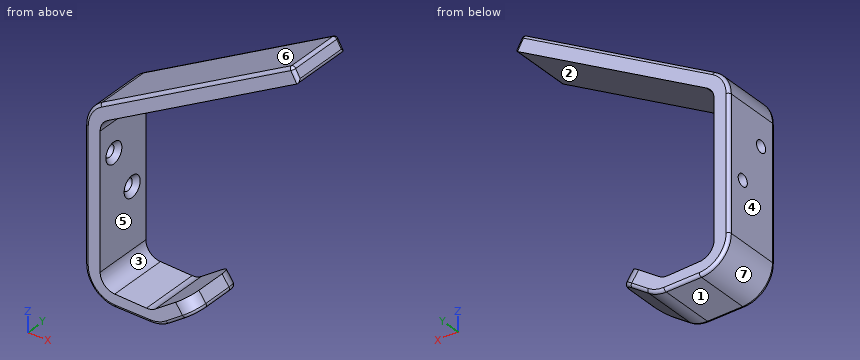
from build123d import *

# Parameters (mm, degrees)
F1_DEPTH       = 20
F2_R           = 10
F3_R           = 10
F4_R           = 5
F5_R           = 5
F6_R           = 5
F8_D           = 4
F8_DEPTH       = 12
F8_CSINK_D     = 7
F8_CSINK_ANGLE = 90
F8_TIP         = 1.2017212381
F9_T1_DEPTH    = 30.0048285071
F10_R          = 1
F11_T1_DEPTH   = 25
F11_T3_DEPTH   = 18
F11_T5_DEPTH   = 6.5
F11_T8_ANGLE   = 90
F11_T10_ANGLE  = 90


# Not quite as in the source:
# - a fillet or chamfer that OpenCascade refuses, or shapes differently, is made with other operations: its cross-section is extruded or revolved along the edge and cut away or added


with BuildPart() as f1:
    # F0 (on Front) → F1 (new body)
    with BuildSketch(Plane.XZ):
        Polygon((13.3003787555, -46.1032405242), (38.3003787555, -46.1032405242), (50.5316518247, -37.4287553132), (47.6391971652, -33.3503112419), (35.4933471628, -41.9642139506), (18.3003787555, -41.5471586402), (18.3003787555, 11.0100081298), (85.0824110582, 49.5666324568), (82.5824110582, 53.8967594758), (13.3003787555, 13.8967594758), align=None)
    extrude(amount=F1_DEPTH)

    # F2
    f2_edges = [f1.edges().sort_by_distance(p)[0] for p in [
        (13.300379, -10, 13.896759),
        (13.300379, -10, -46.103241),
    ]]
    fillet(f2_edges, radius=F2_R)

    # F3
    f3_edges = [f1.edges().sort_by_distance(p)[0] for p in [
        (38.300379, -10, -46.103241),
    ]]
    fillet(f3_edges, radius=F3_R)

    # F4
    f4_edges = [f1.edges().sort_by_distance(p)[0] for p in [
        (18.300379, -10, 11.010008),
    ]]
    fillet(f4_edges, radius=F4_R)

    # F5
    f5_edges = [f1.edges().sort_by_distance(p)[0] for p in [
        (18.300379, -10, -41.547159),
    ]]
    fillet(f5_edges, radius=F5_R)

    # F6
    f6_edges = [f1.edges().sort_by_distance(p)[0] for p in [
        (35.493347, -10, -41.964214),
    ]]
    fillet(f6_edges, radius=F6_R)

    # F8
    with Locations(Plane.YZ.offset(18.3003787555)):
        with Locations((-6, -16.6669744052), (-14, -1.8767432161)):
            CounterSinkHole(F8_D / 2, F8_CSINK_D / 2, depth=F8_DEPTH, counter_sink_angle=F8_CSINK_ANGLE)
            with Locations((0, 0, -(F8_DEPTH + F8_TIP / 2))):  # 118° drill point
                Cone(0, F8_D / 2, F8_TIP, mode=Mode.SUBTRACT)

    # F9: fillet of radius 5 on 2 edges, made by hand

    # F9_s2 → F9_t1 (cut)
    with BuildSketch(Plane(origin=(41.804493112, 0, -58.9455349028), x_dir=(0, 1, 0), z_dir=(-0.5784909319, 0, 0.8156888143))):
        with BuildLine():
            ThreePointArc((0.0004, -14.5649419331), (-1.4644660941, -18.1014415245), (-5.0009656854, -19.5663076185))
            Line((-5.0009656854, -19.5663076185), (-5.0009656854, -20.0664441871))
            ThreePointArc((-5.0009656854, -20.0664441871), (-2.5004828427, -20.0660441871), (0, -20.0660441871))
            Line((0, -20.0660441871), (0.5001365685, -19.5659076185))
            ThreePointArc((0.5001365685, -19.5659076185), (0.5001365685, -17.0654247758), (0.5005365685, -14.5649419331))
            Line((0.5005365685, -14.5649419331), (0.0004, -14.5649419331))
        make_face()
        with BuildLine():
            ThreePointArc((-14.9990343146, -19.5663076185), (-18.5355339059, -18.1014415245), (-20.0004, -14.5649419331))
            Line((-20.0004, -14.5649419331), (-20.5005365685, -14.5649419331))
            ThreePointArc((-20.5005365685, -14.5649419331), (-20.5001365685, -17.0654247758), (-20.5001365685, -19.5659076185))
            Line((-20.5001365685, -19.5659076185), (-20, -20.0660441871))
            ThreePointArc((-20, -20.0660441871), (-17.4995171573, -20.0660441871), (-14.9990343146, -20.0664441871))
            Line((-14.9990343146, -20.0664441871), (-14.9990343146, -19.5663076185))
        make_face()
    extrude(amount=F9_T1_DEPTH, mode=Mode.SUBTRACT)

    # F10
    f10_edges = [f1.edges().sort_by_distance(p)[0] for p in [
        (50.441395, -20, 35.340135),
        (14.640125, -20, 13.123257),
        (13.300379, -20, -13.989992),
        (16.229311, -20, -43.174308),
        (29.207344, -20, -46.103241),
        (38.150024, -20, -45.631327),
        (43.701617, -20, -42.272653),
    ]]
    fillet(f10_edges, radius=F10_R)

    # F11: fillet of radius 1 on 6 edges, made by hand

    # F11_s2 → F11_t1 (cut)
    with BuildSketch(Plane.XZ.offset(-2.5)):
        with BuildLine():
            ThreePointArc((84.2163856545, 49.0666324568), (84.6823114807, 49.6738388155), (84.5824110582, 50.4326578606))
            Line((84.5824110582, 50.4326578606), (85.0824110582, 49.5666324568))
            Line((85.0824110582, 49.5666324568), (84.2163856545, 49.0666324568))
        make_face()
    extrude(amount=F11_T1_DEPTH, mode=Mode.SUBTRACT)

    # F11_s4 → F11_t3 (cut)
    with BuildSketch(Plane.XZ.offset(1)):
        with BuildLine():
            ThreePointArc((83.0824110582, 53.030734072), (82.4752046996, 53.4966598983), (81.7163856545, 53.3967594758))
            Line((81.7163856545, 53.3967594758), (82.5824110582, 53.8967594758))
            Line((82.5824110582, 53.8967594758), (83.0824110582, 53.030734072))
        make_face()
    extrude(amount=F11_T3_DEPTH, mode=Mode.SUBTRACT)

    # F11_s6 → F11_t5 (cut)
    with BuildSketch(Plane(origin=(1.0576213207, 0, -1.8318538627), x_dir=(0, 1, 0), z_dir=(-0.5, 0, 0.8660254038))):
        with BuildLine():
            ThreePointArc((0, -97.4668456201), (-0.2928932188, -98.1739524013), (-1, -98.4668456201))
            Line((-1, -98.4668456201), (0, -98.4668456201))
            Line((0, -98.4668456201), (0, -97.4668456201))
        make_face()
        with BuildLine():
            ThreePointArc((-19, -98.4668456201), (-19.7071067812, -98.1739524013), (-20, -97.4668456201))
            Line((-20, -97.4668456201), (-20, -98.4668456201))
            Line((-20, -98.4668456201), (-19, -98.4668456201))
        make_face()
    extrude(amount=F11_T5_DEPTH, mode=Mode.SUBTRACT)

    # F11_s7 → F11_t8 (revolve, cut)
    with BuildSketch(Plane.XZ.offset(1)):
        with BuildLine():
            ThreePointArc((81.7163856545, 53.3967594758), (82.4752046996, 53.4966598983), (83.0824110582, 53.030734072))
            Line((83.0824110582, 53.030734072), (82.5824110582, 53.8967594758))
            Line((82.5824110582, 53.8967594758), (81.7163856545, 53.3967594758))
        make_face()
    revolve(axis=Axis((83.0824110582, -1, 53.030734072), (-0.8660254038, 0, -0.5)), revolution_arc=F11_T8_ANGLE, mode=Mode.SUBTRACT)

    # F11_s9 → F11_t10 (revolve, cut)
    with BuildSketch(Plane.XZ.offset(19)):
        with BuildLine():
            ThreePointArc((83.0824110582, 53.030734072), (82.4752046996, 53.4966598983), (81.7163856545, 53.3967594758))
            Line((81.7163856545, 53.3967594758), (82.5824110582, 53.8967594758))
            Line((82.5824110582, 53.8967594758), (83.0824110582, 53.030734072))
        make_face()
    revolve(axis=Axis((83.0824110582, -19, 53.030734072), (0.8660254038, 0, 0.5)), revolution_arc=F11_T10_ANGLE, mode=Mode.SUBTRACT)


solid = f1.part
The listing builds one solid part. Answer for the finished solid, in the listing's coordinates (mm). Face numbers are marked on the shaded views. A direction names the side the tool comes from. Coordinates: 2 decimals unless noted, no trailing zeros. Write each loop counter-clockwise with the first axis right and the second up, starting at its lowest first coordinate (ties: lowest second). Pieces come first, ordered by that corner, then holes. Notation, with made-up numbers: (27, 50.5) - (46, 50.5) arc R25 ccw to (46, 65.5) - close; hole circle Ø2 at (1, -1.5). An arc over 180 degrees is marked (long way). Return JSON: item names as keys, results as strings.
1. The part is cut by section B-B on z = 6. Determine the outline of the cut face in (x, y), then the cut area to 3 significant figures.
Final values:
{"outline": "(13.3, -19) arc R1 ccw to (14.3, -20) - (18.3, -20) - (18.3, 0) - (14.3, 0) arc R1 ccw to (13.3, -1) - close", "area": "99.6 mm^2"}
2. Each of these flat-tipped pins is pushed along its axis until it touches: pin 1 Ø3.5 at (y, z) = (-14, -1.88) entering from +X; pin 2 Ø12 at (x, y) = (51, -13.5) entering from +Z; pin 3 Ø2 at (y, z) = (-8.5, 40.5) entering from +X; pin 4 Ø6 at (x, y) = (70.5, -5) entering from +Z. Where does it stop, or does it pass through?
Final values:
{"pin 1": "through", "pin 2": "z = 39.13", "pin 3": "x = 71.11", "pin 4": "z = 48.65"}
3. For a pull along Z with two mould halves and no side action, classify the marked faces 4, 5, 6 and 7 as +Z half, -Z half, draft (parallel to the pull), parting line (faces both ways), or undercut.
Final values:
{"face 4": "draft", "face 5": "undercut", "face 6": "+Z half", "face 7": "-Z half"}
4. Which of the six approach directions +Z, -Z, +X, -X, +Y, -Y give full straight-line access (tool end or side, diameter ignored) to the marked faces 1, 2 and 3?
Final values:
{"face 1": "-Z, +X, -X, +Y, -Y", "face 2": "+X, +Y, -Y", "face 3": "+Y, -Y"}
5. Consider line 1 along Z through (x, y) = (15.8, -6); line 2 along Z through (x, y) = (21, -10.5); line 3 along X through (y, z) = (-15.25, -11.5). Determine where each line is inside the solid, lowest interval first.
Final values:
{"line 1": "-42.72 to -18.67, -14.67 to 14.74", "line 2": "-45.84 to -41.11, 12.57 to 18.34", "line 3": "13.3 to 18.3"}
6. The part is cut by section A-A on y = -14. Determine the outline of the cut face in (x, z) (1 decimal), then the cut area to 3 significant figures.
Final values:
{"outline": "(13.3, -36.1) arc R10 ccw to (23.3, -46.1) - (35.1, -46.1) arc R10 ccw to (40.9, -44.3) - (49.7, -38) arc R1 ccw to (50, -36.6) - (47.6, -33.4) - (36.8, -41) arc R5 cw to (33.8, -41.9) - (23.2, -41.7) arc R5 cw to (18.3, -36.7) - (18.3, -5.4) - (16.8, -3.9) - (13.3, -3.9) - close; (13.3, 0.1) - (16.8, 0.1) - (18.3, 1.6) - (18.3, 8.1) arc R5 cw to (20.8, 12.5) - (84.2, 49.1) arc R1 ccw to (84.6, 50.4) - (83.1, 53) arc R1 ccw to (81.7, 53.4) - (18.3, 16.8) arc R10 ccw to (13.3, 8.1) - close", "area": "797 mm^2"}
